Source: three-view drawing plus pictorial views. Frame: mm from the lowest corner of the part. Round coordinates to 2 decimals unless told otherwise and drop trailing zeros. Loops run counter-clockwise (first coordinate to the right, second up) from the corner with the lowest first, then second, coordinate; pieces in that order, holes last. Notation, with made-up numbers: (42.25, -17.5) -> (56.25, -17.5) arc R31 cw to (56.25, 8.5) -> close; hole circle Ø8 at (12, 70). An arc over 180 degrees is marked (long way). One line per question, with ' | ' between items. Start each with the question number.
Q1. Material intervals for L1, parallel to X at y = 61.5, z = 6.75; L2, parallel to X at y = 35, z = 1.5; L3, parallel to X at y = 112, z = 0.75, sorted ascending.
Q2. Cut plane A-A on x = 45. Return loops of the section in (y, z).
Q3. Cut plane C-C on y = 23. Return loops of the section in (x, z).
Q4. Cut plane B-B on z = 3.75. Return loops of the section in (x, y).
Q5. Contact query for a flat-ended pin moving along its axis: P1, Ø5, axis at x = 34, y = 18.5, coming from the +Z side. Output: stop coordinate, or through.
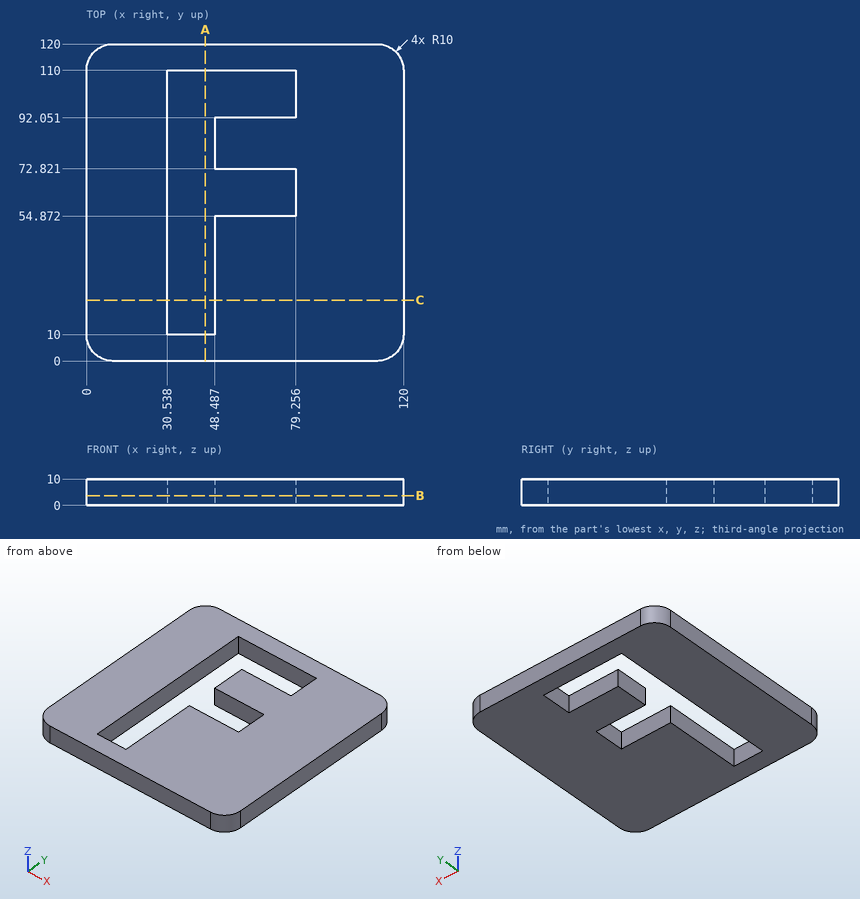
Results:
1) L1: 0 to 30.54, 79.26 to 120 | L2: 0 to 30.54, 48.49 to 120 | L3: 0.2 to 119.8
2) outline: (0, 0) -> (10, 0) -> (10, 10) -> (0, 10) -> close; (110, 0) -> (120, 0) -> (120, 10) -> (110, 10) -> close
3) outline: (0, 0) -> (30.54, 0) -> (30.54, 10) -> (0, 10) -> close; (48.49, 0) -> (120, 0) -> (120, 10) -> (48.49, 10) -> close
4) outline: (0, 10) arc R10 ccw to (10, 0) -> (110, 0) arc R10 ccw to (120, 10) -> (120, 110) arc R10 ccw to (110, 120) -> (10, 120) arc R10 ccw to (0, 110) -> close; hole (30.54, 10) -> (48.49, 10) -> (48.49, 54.87) -> (79.26, 54.87) -> (79.26, 72.82) -> (48.49, 72.82) -> (48.49, 92.05) -> (79.26, 92.05) -> (79.26, 110) -> (30.54, 110) -> close
5) P1: through
